```python
from build123d import *

# Parameters (mm, degrees)
BOSS_EXTRUDE1_DEPTH                           = 10
BOSS_EXTRUDE2_DEPTH                           = 40
CBORE_FOR_M6_CHEESE_SLOTTED_HEAD1_D           = 6.4
CBORE_FOR_M6_CHEESE_SLOTTED_HEAD1_DEPTH       = 15
CBORE_FOR_M6_CHEESE_SLOTTED_HEAD1_CBORE_D     = 11
CBORE_FOR_M6_CHEESE_SLOTTED_HEAD1_CBORE_DEPTH = 3.9
MIRROR4_COPY_1_D                              = 6.4
MIRROR4_COPY_1_DEPTH                          = 15
MIRROR4_COPY_1_CBORE_D                        = 11
MIRROR4_COPY_1_CBORE_DEPTH                    = 3.9
FILLET1_R                                     = 10
FILLET2_R                                     = 15
FILLET3_R                                     = 10
FILLET4_R                                     = 15
FILLET5_R                                     = 1
SKETCH5_R                                     = 35
CUT_EXTRUDE1_DEPTH                            = 61
FILLET6_R                                     = 2


with BuildPart() as part:
    # Sketch1 → Boss-Extrude1 (new body, symmetric)
    with BuildSketch(Plane.XY):
        with BuildLine():
            Line((-100, -60), (100, -60))
            Line((100, -60), (100, -45))
            Line((100, -45), (90.015821042, -45))
            Line((90.015821042, -45), (41.622765631, 27.704609385))
            ThreePointArc((41.622765631, 27.704609385), (0, 50), (-41.622765631, 27.704609385))
            Line((-41.622765631, 27.704609385), (-90.015821042, -45))
            Line((-90.015821042, -45), (-100, -45))
            Line((-100, -45), (-100, -60))
        make_face()
    extrude(amount=BOSS_EXTRUDE1_DEPTH, both=True)

    # Sketch2 → Boss-Extrude2 (add)
    with BuildSketch(Plane.XY.offset(10)):
        Polygon((90.015821042, -45), (60, -45), (60, -60), (100, -60), (100, -45), align=None)
        Polygon((-60, -60), (-60, -45), (-90.015821042, -45), (-100, -45), (-100, -60), align=None)
    boss_extrude2 = extrude(amount=BOSS_EXTRUDE2_DEPTH)

    # Mirror2: Boss-Extrude2 across plane
    add(boss_extrude2.mirror(Plane.XY))

    # CBORE for M6 Cheese Slotted Head1
    with Locations(Plane(origin=(80, -45, -30), x_dir=(0, 0, 1), z_dir=(0, 1, 0))):
        with Locations((0, 0)):
            cbore_for_m6_cheese_slotted_head1 = CounterBoreHole(CBORE_FOR_M6_CHEESE_SLOTTED_HEAD1_D / 2, CBORE_FOR_M6_CHEESE_SLOTTED_HEAD1_CBORE_D / 2, CBORE_FOR_M6_CHEESE_SLOTTED_HEAD1_CBORE_DEPTH, depth=CBORE_FOR_M6_CHEESE_SLOTTED_HEAD1_DEPTH)

    # Mirror3: CBORE for M6 Cheese Slotted Head1 across plane
    add(cbore_for_m6_cheese_slotted_head1.mirror(Plane(origin=(0, 0, 0), x_dir=(0, 0, 1), z_dir=(1, 0, 0))), mode=Mode.SUBTRACT)

    # Mirror4: CBORE for M6 Cheese Slotted Head1 across plane
    add(cbore_for_m6_cheese_slotted_head1.mirror(Plane.XY), mode=Mode.SUBTRACT)

    # Mirror4 copy 1
    with Locations(Plane(origin=(-80, -45, 30), x_dir=(0, 0, -1), z_dir=(0, 1, 0))):
        with Locations((0, 0)):
            CounterBoreHole(MIRROR4_COPY_1_D / 2, MIRROR4_COPY_1_CBORE_D / 2, MIRROR4_COPY_1_CBORE_DEPTH, depth=MIRROR4_COPY_1_DEPTH)

    # Fillet1
    fillet1_edges = [part.edges().sort_by_distance(p)[0] for p in [
        (90.015821042, -45, 0),
        (60, -52.5, 10),
        (75.007910521, -45, 10),
        (75.007910521, -45, -10),
        (60, -52.5, -10),
    ]]
    fillet(fillet1_edges, radius=FILLET1_R)

    # Fillet2
    fillet2_edges = [part.edges().sort_by_distance(p)[0] for p in [
        (60, -52.5, 50),
        (100, -52.5, 50),
        (100, -52.5, -50),
        (60, -52.5, -50),
    ]]
    fillet(fillet2_edges, radius=FILLET2_R)

    # Fillet3
    fillet3_edges = [part.edges().sort_by_distance(p)[0] for p in [
        (-90.015821042, -45, 0),
        (-75.007910521, -45, 10),
        (-60, -52.5, 10),
        (-75.007910521, -45, -10),
        (-60, -52.5, -10),
    ]]
    fillet(fillet3_edges, radius=FILLET3_R)

    # Fillet4
    fillet4_edges = [part.edges().sort_by_distance(p)[0] for p in [
        (-60, -52.5, 50),
        (-100, -52.5, 50),
        (-100, -52.5, -50),
        (-60, -52.5, -50),
    ]]
    fillet(fillet4_edges, radius=FILLET4_R)

    # Fillet5
    fillet5_edges = [part.edges().sort_by_distance(p)[0] for p in [
        (62.491233684, -3.647695307, 10),
        (62.491233684, -3.647695307, -10),
        (85.262771791, -37.85912852, 10.417443759),
        (85.262771791, -37.85912852, -10.417443759),
        (90.886474153, -43.93738446, -15.514115582),
        (90.886474153, -43.93738446, 15.514115582),
        (-85.262771791, -37.85912852, 10.417443759),
        (-85.262771791, -37.85912852, -10.417443759),
        (-90.886474153, -43.93738446, 15.514115582),
        (-90.886474153, -43.93738446, -15.514115582),
        (0, 50, 10),
        (-62.491233684, -3.647695307, 10),
        (-62.491233684, -3.647695307, -10),
        (0, 50, -10),
    ]]
    fillet(fillet5_edges, radius=FILLET5_R)

    # Sketch5 → Cut-Extrude1 (cut, through all)
    with BuildSketch(Plane(origin=(0, 0, -10), x_dir=(-1, 0, 0), z_dir=(0, 0, -1))):
        Circle(SKETCH5_R)
    extrude(amount=-CUT_EXTRUDE1_DEPTH, mode=Mode.SUBTRACT)

    # Fillet6
    fillet6_edges = [part.edges().sort_by_distance(p)[0] for p in [
        (35, 0, 10),
        (35, 0, -10),
    ]]
    fillet(fillet6_edges, radius=FILLET6_R)


solid = part.part
```
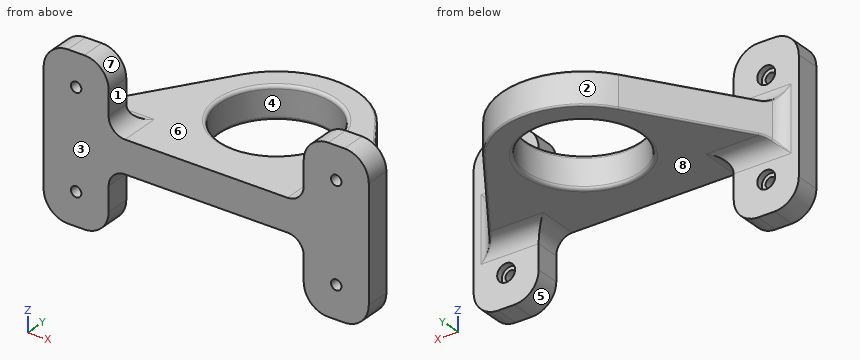
Source: CAD feature listing. Evaluate the final solid. Frame: model axes, mm. Face numbers are marked on the shaded views. A direction names the side the tool comes from. Coordinates: 2 decimals unless noted, no trailing zeros. Loops run counter-clockwise (first coordinate to the right, second up) from the corner with the lowest first, then second, coordinate; pieces in that order, holes last. Notation, with made-up numbers: (-14, 58) -> (23, 58) arc R26 cw to (23, 93) -> close; hole circle Ø7 at (15.5, 89.5). An arc over 180 degrees is marked (long way). One line per item, written item: value. Start each with the question number.
Q1. Section query D-D, the plane z = -40. Return the cut outline in (x, y), and give its area (3 significant figures).
Q2. Mould query, pull axis Y, two halves, no side actions, for the marked faces 1, 2, 3 and 4. Classes: pulls with the +Y half, pulls with the -Y half, needs draft (parallel to the pull), parting line crosses it, or undercut.
Q3. Section query A-A, the plane z = -30. Return the cut outline in (x, y).
Q4. Section query B-B, the plane x = 0. Return the cut outline in (y, z), and give its area (3 significant figures).
Q5. Set-up query: the marked faces 5, 6, 7 and 8. Return all of +Z, -Z, +X, -X, +Y, -Y with unobstructed straight access to the full face (end or side cutting, diameter ignored); none if empty.
Q6. Section query C-C, the plane z = -5. Return the cut outline in (x, y).
Q7. Contact query for flat-ended pins moving along their axis: P1, Ø12, axis at x = 79, z = -31.5, coming from the +Y side; P2, Ø20, axis at x = 88, z = 8.5, coming from the +Y side; P3, Ø6, axis at x = 80, z = -30, coming from the +Y side; P4, Ø14.5, axis at x = -80, z = -30, coming from the -Y side. Output: stop coordinate, or through.
Q8. Line query: line 1 along X through (y, z) = (-47, 30); line 2 along Z through (x, y) = (-80, -46.65); line 3 along X through (y, z) = (-52, -23). Output: solid intervals per line, ascending.
Results:
1. outline: (-99.14, -60) -> (-60.86, -60) -> (-60.86, -45) -> (-99.14, -45) -> close; (60.86, -60) -> (99.14, -60) -> (99.14, -45) -> (60.86, -45) -> close
1. area: 1,150 mm^2
2. face 1: needs draft
2. face 2: pulls with the +Y half
2. face 3: pulls with the -Y half
2. face 4: undercut
3. outline: (-100, -60) -> (-83.2, -60) -> (-83.2, -48.9) -> (-85.5, -48.9) -> (-85.5, -45) -> (-100, -45) -> close; (-76.8, -60) -> (-60, -60) -> (-60, -45) -> (-74.5, -45) -> (-74.5, -48.9) -> (-76.8, -48.9) -> close; (60, -60) -> (76.8, -60) -> (76.8, -48.9) -> (74.5, -48.9) -> (74.5, -45) -> (60, -45) -> close; (83.2, -60) -> (100, -60) -> (100, -45) -> (85.5, -45) -> (85.5, -48.9) -> (83.2, -48.9) -> close
4. outline: (-60, -10) -> (-37, -10) arc R2 ccw to (-35, -8) -> (-35, 8) arc R2 ccw to (-37, 10) -> (-60, 10) -> close; (35, -8) arc R2 ccw to (37, -10) -> (49, -10) arc R1 ccw to (50, -9) -> (50, 9) arc R1 ccw to (49, 10) -> (37, 10) arc R2 ccw to (35, 8) -> close
4. area: 796 mm^2
5. face 5: -Z, +Y, -Y
5. face 6: +Z, +Y
5. face 7: +Z, +Y, -Y
5. face 8: -Z, +Y
6. outline: (-100, -60) -> (100, -60) -> (100, -45) -> (95.37, -45) arc R10 cw to (87.05, -40.54) -> (41.62, 27.7) arc R50 ccw to (-41.62, 27.7) -> (-87.05, -40.54) arc R10 cw to (-95.37, -45) -> (-100, -45) -> close; hole circle Ø70 at (0, 0)
7. P1: y = -45
7. P2: y = -26.95
7. P3: through
7. P4: y = -60
8. line 1: -100 to -85.5, -74.5 to -60, 60 to 74.5, 85.5 to 100
8. line 2: -50 to -35.5, -24.5 to 24.5, 35.5 to 50
8. line 3: -100 to -60, 60 to 100
